The drawing under review shows one solid part. Ordinate dimensions are in mm from its lowest x, y, z. A direction names the side the tool comes from. Coordinates: 2 decimals unless noted, no trailing zeros. Write each loop counter-clockwise with the first axis right and the second up, starting at its lowest first coordinate (ties: lowest second). Pieces come first, ordered by that corner, then holes.
1) We need section D-D on y = 21. Write out the cut boundary in (x, z), then the cut area to 3 significant figures.
2) Insertion check: P1, Ø1, axis at x = 40.5, y = 15.5, coming from the +Z side; P2, Ø0.8, axis at y = 32.5, z = 12, coming from the -X side; P3, Ø1.1, axis at y = 0.5, z = 14, coming from the -X side; P4, Ø0.8, axis at y = 32.5, z = 13, coming from the +X side. Each pin has a flat end and moves straight along its axis. Give the tip position at first contact, or say it passes through.
3) We need section C-C on z = 6.5. Write out the cut boundary in (x, y).
4) To check wall thickness, follow line 1 along X through (y, z) = (16.5, 10); line 2 along Y through (x, z) = (29, 16); line 3 along X through (y, z) = (24, 14.75). State the ranges of each line that lie inside material, in increasing order.
5) We need section B-B on x = 14. Write out the cut boundary in (y, z), then the cut area to 3 significant figures.
6) Mouldability with a two-part tool opening along Y and no side actions: class the marked faces 3, 4 and 5 as pulls with the +Y half, pulls with the -Y half, needs draft (parallel to the pull), parting line crosses it, or undercut.
7) For the marked faces 1 and 2, list the 3-axis set-ups (+Z, -Z, +X, -X, +Y, -Y) from which the entire face can be reached by the end or side of a thin tool; tool diameter is ignored.
8) We need section A-A on z = 12. Write out the cut boundary in (x, y), then the cut area to 3 significant figures.
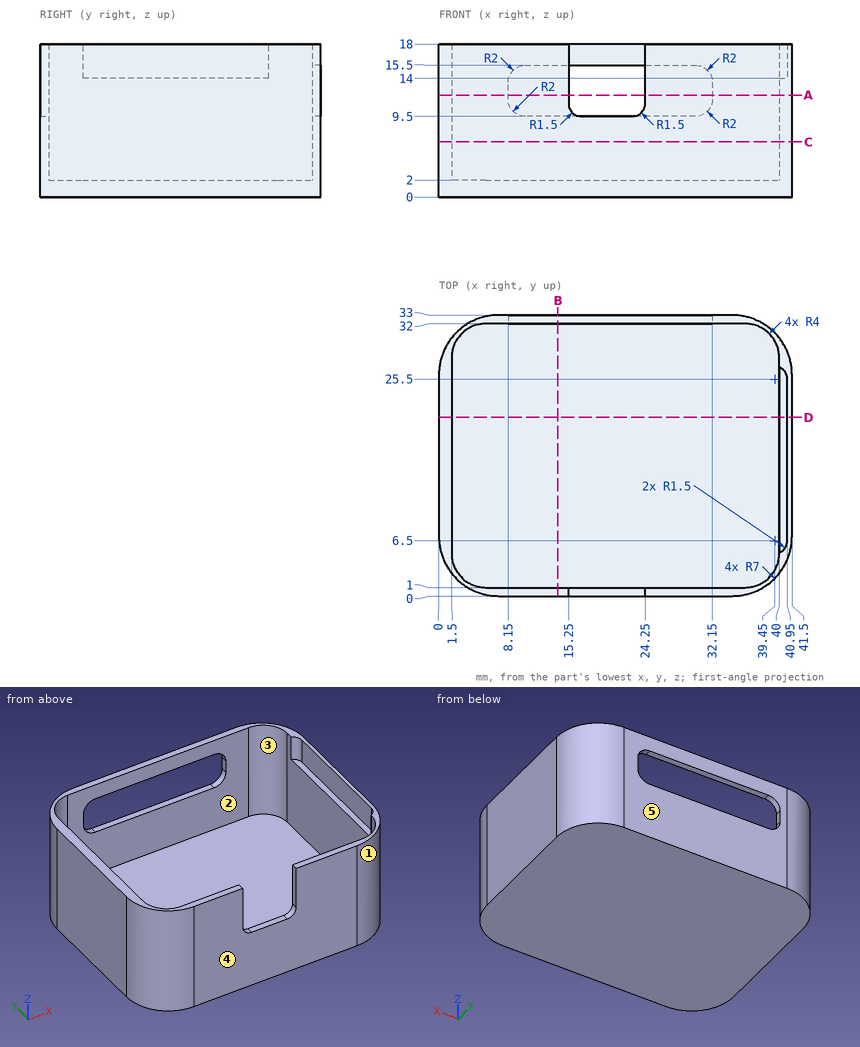
Result:
1. outline: (0, 0) - (41.5, 0) - (41.5, 18) - (40.95, 18) - (40.95, 14) - (40, 14) - (40, 2) - (1.5, 2) - (1.5, 18) - (0, 18) - close
1. area: 127 mm2
2. P1: stops at z = 18
2. P2: stops at x = 3.57
2. P3: stops at x = 3.31
2. P4: stops at x = 37.93
3. outline: (0, 7) arc R7 ccw to (7, 0) - (34.5, 0) arc R7 ccw to (41.5, 7) - (41.5, 26) arc R7 ccw to (34.5, 33) - (7, 33) arc R7 ccw to (0, 26) - close; hole (1.5, 5) arc R4 ccw to (5.5, 1) - (36, 1) arc R4 ccw to (40, 5) - (40, 28) arc R4 ccw to (36, 32) - (5.5, 32) arc R4 ccw to (1.5, 28) - close
4. line 1: x = 0 to 1.5, 40 to 41.5
4. line 2: y = 0 to 1, 32 to 33
4. line 3: x = 0 to 1.5, 40.95 to 41.5
5. outline: (0, 0) - (33, 0) - (33, 9.5) - (32, 9.5) - (32, 2) - (1, 2) - (1, 18) - (0, 18) - close; (32, 15.5) - (33, 15.5) - (33, 18) - (32, 18) - close
5. area: 92.0 mm2
6. face 3: undercut
6. face 4: pulls with the -Y half
6. face 5: pulls with the +Y half
7. face 1: +Z, -Z, +X, -Y
7. face 2: +Z
8. outline: (0, 7) arc R7 ccw to (7, 0) - (15.25, 0) - (15.25, 1) - (5.5, 1) arc R4 cw to (1.5, 5) - (1.5, 28) arc R4 cw to (5.5, 32) - (8.15, 32) - (8.15, 33) - (7, 33) arc R7 ccw to (0, 26) - close; (24.25, 0) - (34.5, 0) arc R7 ccw to (41.5, 7) - (41.5, 26) arc R7 ccw to (34.5, 33) - (32.15, 33) - (32.15, 32) - (36, 32) arc R4 cw to (40, 28) - (40, 5) arc R4 cw to (36, 1) - (24.25, 1) - close
8. area: 115 mm2
